Source: CAD feature listing. Evaluate the final solid. Frame: model axes, mm. A direction names the side the tool comes from. Give positions to 0.01 mm unless a question says otherwise; leave off trailing zeros. Loops run counter-clockwise (first coordinate to the right, second up) from the corner with the lowest first, then second, coordinate; pieces in that order, holes last. Notation, with made-up numbers: M -13,42 L 16,42 A19 ccw 16,77 Z; hole C 35,54.5 d11. An arc over 180 degrees is marked long. Put each result on its own line as item: value.
from build123d import *

# Parameters (mm, degrees)
SKETCH1_R           = 1.75
SKETCH1_R_2         = 5
BOSS_EXTRUDE1_DEPTH = 10


with BuildPart() as part:
    # Sketch1 → Boss-Extrude1 (new body)
    with BuildSketch(Plane.XY):
        with BuildLine():
            Line((59.115327383, 43.551262968), (93.822811009, 43.551262968))
            ThreePointArc((93.822811009, 43.551262968), (97.822811009, 39.551262968), (93.822811009, 35.551262968))
            Line((93.822811009, 35.551262968), (73.221068218, 35.551262968))
            ThreePointArc((73.221068218, 35.551262968), (65.430500205, 30.870379763), (65.905746743, 21.794160382))
            ThreePointArc((65.905746743, 21.794160382), (67.305407589, 18.859363547), (67.785956814, 15.64359686))
            Line((67.785956814, 15.64359686), (67.785956814, 7.945306105))
            ThreePointArc((67.785956814, 7.945306105), (67.117243875, 5.990433735), (65.715264602, 4.47281814))
            ThreePointArc((65.715264602, 4.47281814), (62.263505272, 3.582643734), (59.096031047, 5.217929635))
            ThreePointArc((59.096031047, 5.217929635), (55.724954026, 7.67997226), (51.642471122, 8.551262968))
            Line((51.642471122, 8.551262968), (46.626949913, 8.551262968))
            ThreePointArc((46.626949913, 8.551262968), (39.555882101, 11.480195156), (36.626949913, 18.551262968))
            Line((36.626949913, 18.551262968), (36.626949913, 38.848632096))
            ThreePointArc((36.626949913, 38.848632096), (42.251881835, 47.568318218), (52.515088487, 46.03881686))
            ThreePointArc((52.515088487, 46.03881686), (55.588605185, 44.19379373), (59.115327383, 43.551262968))
        make_face()
        with Locations((93.822811009, 39.551262968)):
            Circle(SKETCH1_R, mode=Mode.SUBTRACT)
        with Locations((62.822811009, 39.551262968)):
            Circle(SKETCH1_R, mode=Mode.SUBTRACT)
        with Locations((62.822811009, 8.551262968)):
            Circle(SKETCH1_R, mode=Mode.SUBTRACT)
        with Locations((45.725055781, 39.551262968)):
            Circle(SKETCH1_R_2, mode=Mode.SUBTRACT)
        with Locations((45.725055781, 17.551264875)):
            Circle(SKETCH1_R_2, mode=Mode.SUBTRACT)
    extrude(amount=-BOSS_EXTRUDE1_DEPTH)


solid = part.part
1. Section query B-B (y = 16.5). Output: boundary loops of the cut face in (x, z), plus the area to 3 significant figures.
Found:
outline: M 36.84,-10 L 40.84,-10 L 40.84,0 L 36.84,0 Z; M 50.61,-10 L 67.75,-10 L 67.75,0 L 50.61,0 Z
area: 211 mm^2
2. Section query C-C (x = 94.5). Output: boundary loops of the cut face in (y, z).
Found:
outline: M 35.61,-10 L 37.94,-10 L 37.94,0 L 35.61,0 Z; M 41.16,-10 L 43.49,-10 L 43.49,0 L 41.16,0 Z
3. Contact query for flat-ended pins moving along their axis: P1, Ø1, axis at y = 13.5, z = -7.5, coming from the -X side; P2, Ø4, axis at x = 49.5, z = -3.5, coming from the -Y side; P3, Ø2, axis at x = 87, z = -8.5, coming from the -Y side; P4, Ø16, axis at x = 45.73, y = 39.55, coming from the +Z side. Output: stop coordinate, or through.
Found:
P1: x = 37.72
P2: y = 8.55
P3: y = 35.55
P4: z = 0
4. Section query A-A (x = 42). Output: boundary loops of the cut face in (y, z), plus the area to 3 significant figures.
Found:
outline: M 9.69,-10 L 14.22,-10 L 14.22,0 L 9.69,0 Z; M 20.89,-10 L 36.22,-10 L 36.22,0 L 20.89,0 Z; M 42.89,-10 L 47.45,-10 L 47.45,0 L 42.89,0 Z
area: 244 mm^2
5. Material intervals for line 1 (X direction, y = 38, z = -6.75); line 2 (Y direction, x = 45, z = -7.5); line 3 (Y direction, x = 75, z = -1.75), sorted ascending. Write a range as from..to.
Found:
line 1: 36.63..40.97, 50.48..62.01, 63.63..93.01, 94.63..97.51
line 2: 8.68..12.6, 22.5..34.6, 44.5..48.34
line 3: 35.55..43.55
6. Access query for faces 4 (the flat face through (76, 43.551, -5)), 5 (the flat face through (67.786, 12, -5)), 6 (the cylindrical face through (97.82, 39.64, -4.93)), 7 (the flat face through (49, 8.551, -5)), 8 (the flat face through (36.627, 29, -5)). Directions: +Z, -Z, +X, -X, +Y, -Y. A direction counts if a zero-diameter tool reaches every point of the face in a straight line with its end or side. Return the directions, or none.
Found:
face 4: +Z, -Z, +X, +Y
face 5: +Z, -Z, +X, -Y
face 6: +Z, -Z, +X
face 7: +Z, -Z, -X, -Y
face 8: +Z, -Z, -X, +Y, -Y
7. Section query D-D (z = -5.5). Output: boundary loops of the cut face in (x, y), plus the area to 3 significant figures.
Found:
outline: M 36.63,18.55 A10 ccw 46.63,8.55 L 51.64,8.55 A10 cw 59.1,5.22 A5 ccw 67.79,7.95 L 67.79,15.64 A11 ccw 65.91,21.79 A8.82 cw 73.22,35.55 L 93.82,35.55 A4 ccw 93.82,43.55 L 59.12,43.55 A10 cw 52.52,46.04 A9.57 ccw 36.63,38.85 Z; hole C 45.73,17.55 d10; hole C 45.73,39.55 d10; hole C 62.82,8.55 d3.5; hole C 62.82,39.55 d3.5; hole C 93.82,39.55 d3.5
area: 1,190 mm^2
8. Draft query along Y for faces 1 (the flat face through (84, 35.551, -5)), 2 (the cylindrical face through (41.757, 14.509, -4.93)), 3 (the cylindrical face through (42.1, 47.5, -4.9)). Return one class per face: pulls with the +Y half, pulls with the -Y half, needs draft (parallel to the pull), parting line crosses it, or undercut.
Found:
face 1: pulls with the -Y half
face 2: undercut
face 3: pulls with the +Y half
